from build123d import *

# Parameters (mm, degrees)
EA_RSA40X40X5_1_DEPTH = 360


with BuildPart() as part:
    # Sketch1 → Ea RSA40X40X5(1) (new body)
    with BuildSketch(Plane.XY.offset(-180)):
        with BuildLine():
            Line((0, 90), (0, 0))
            Line((0, 0), (150, 0))
            Line((150, 0), (150, 9))
            ThreePointArc((150, 9), (148.242640687, 13.242640687), (144, 15))
            Line((144, 15), (27, 15))
            ThreePointArc((27, 15), (18.514718626, 18.514718626), (15, 27))
            Line((15, 27), (15, 84))
            ThreePointArc((15, 84), (13.242640687, 88.242640687), (9, 90))
            Line((9, 90), (0, 90))
        make_face()
    extrude(amount=EA_RSA40X40X5_1_DEPTH)


solid = part.part
CAD build for the part. Positions are in the model's coordinates, mm. A direction names the side the tool comes from. Give positions to 0.01 mm unless a question says otherwise; leave off trailing zeros. Order: outer loops, then holes, each group sorted by start corner. A loop starts at its lowest first (then second) coordinate and runs counter-clockwise, first axis right, second up. Notation, with made-up numbers: (61.25, -12) - (66.25, -12) arc R19 ccw to (66.25, 8) - close; hole circle Ø9 at (24, 30). An arc over 180 degrees is marked (long way). Write each question's results on one line, items separated by ' | '.
1. Pin check, flat tip, straight feed: pin 1 (4 mm diameter, centred on y = 39.5, z = 8, fed in from +X). Stop position of the tip, or through.
Calculated:
pin 1: stops at x = 15
2. Saw through at A-A on z = 48.5. List the corners of the cut face in (x, y).
Calculated:
outline: (0, 0) - (150, 0) - (150, 9) arc R6 ccw to (144, 15) - (27, 15) arc R12 cw to (15, 27) - (15, 84) arc R6 ccw to (9, 90) - (0, 90) - close
3. Probe L1, parallel to X at y = 9.5, z = -83.5; L2, parallel to X at y = 74.5, z = -75.5. List the from-to ranges inside material, lowest first. Write a range as from..to.
Calculated:
L1: x = 0..149.98 | L2: x = 0..15
4. 3-axis set-ups, long thin cutter, end or side, ignore diameter. For faces 1 (the face through (74, 0, -3)), 2 (the face through (86, 15, -3)): which of +Z, -Z, +X, -X, +Y, -Y reach the whole face in a straight line?
Calculated:
face 1: +Z, -Z, +X, -X, -Y | face 2: +Z, -Z, +X, +Y
5. Saw through at B-B on y = 57. List the corners of the cut face in (x, z).
Calculated:
outline: (0, -180) - (15, -180) - (15, 180) - (0, 180) - close
